```python
from build123d import *

# Parameters (mm, degrees)
SKETCH_1_R          = 45
SKETCH_1_R_2        = 2.6
SKETCH_1_R_3        = 35
EXTRUDE_2_DEPTH     = 5
EXTRUDE_START       = -5
SKETCH_3_R          = 47.8
SKETCH_3_R_2        = 45
EXTRUDE_3_DEPTH     = 5
CUT_EXTRUDE_1_DEPTH = 10


with BuildPart() as part:
    # 草图1 → 凸台-拉伸2 (new body)
    with BuildSketch(Plane.XY):
        Circle(SKETCH_1_R)
        with Locations((0, 40)):
            Circle(SKETCH_1_R_2, mode=Mode.SUBTRACT)
        with Locations((28.284271247, 28.284271247)):
            Circle(SKETCH_1_R_2, mode=Mode.SUBTRACT)
        with Locations((40, 0)):
            Circle(SKETCH_1_R_2, mode=Mode.SUBTRACT)
        with Locations((28.284271247, -28.284271247)):
            Circle(SKETCH_1_R_2, mode=Mode.SUBTRACT)
        with Locations((0, -40)):
            Circle(SKETCH_1_R_2, mode=Mode.SUBTRACT)
        with Locations((-28.284271247, -28.284271247)):
            Circle(SKETCH_1_R_2, mode=Mode.SUBTRACT)
        Circle(SKETCH_1_R_3, mode=Mode.SUBTRACT)
        with Locations((-40, 0)):
            Circle(SKETCH_1_R_2, mode=Mode.SUBTRACT)
        with Locations((-28.284271247, 28.284271247)):
            Circle(SKETCH_1_R_2, mode=Mode.SUBTRACT)
    extrude(amount=EXTRUDE_2_DEPTH)

    # 草图3 → 凸台-拉伸3 (add)
    with BuildSketch(Plane.XY.offset(5).offset(EXTRUDE_START)):
        Circle(SKETCH_3_R)
        Circle(SKETCH_3_R_2, mode=Mode.SUBTRACT)
    extrude(amount=EXTRUDE_3_DEPTH)

    # 草图4 → 切除-拉伸1 (cut)
    with BuildSketch(Plane.XY.offset(5)):
        with BuildLine():
            ThreePointArc((-8.473137213, 41.646799946), (-16.264045876, 39.264880132), (-23.457321876, 35.440147438))
            ThreePointArc((-23.457321876, 35.440147438), (-24.162193968, 31.975590419), (-20.697636949, 31.270718328))
            ThreePointArc((-20.697636949, 31.270718328), (-14.350628714, 34.645482469), (-7.476297541, 36.747176423))
            ThreePointArc((-7.476297541, 36.747176423), (-5.524905615, 39.695408021), (-8.473137213, 41.646799946))
        make_face()
        with BuildLine():
            ThreePointArc((23.457321876, 35.440147438), (16.264045876, 39.264880132), (8.473137213, 41.646799946))
            ThreePointArc((8.473137213, 41.646799946), (5.524905615, 39.695408021), (7.476297541, 36.747176423))
            ThreePointArc((7.476297541, 36.747176423), (14.350628714, 34.645482469), (20.697636949, 31.270718328))
            ThreePointArc((20.697636949, 31.270718328), (24.162193968, 31.975590419), (23.457321876, 35.440147438))
        make_face()
        with BuildLine():
            ThreePointArc((41.646799946, 8.473137213), (39.264880132, 16.264045876), (35.440147438, 23.457321876))
            ThreePointArc((35.440147438, 23.457321876), (31.975590419, 24.162193968), (31.270718328, 20.697636949))
            ThreePointArc((31.270718328, 20.697636949), (34.645482469, 14.350628714), (36.747176423, 7.476297541))
            ThreePointArc((36.747176423, 7.476297541), (39.695408021, 5.524905615), (41.646799946, 8.473137213))
        make_face()
        with BuildLine():
            ThreePointArc((35.440147438, -23.457321876), (39.264880132, -16.264045876), (41.646799946, -8.473137213))
            ThreePointArc((41.646799946, -8.473137213), (39.695408021, -5.524905615), (36.747176423, -7.476297541))
            ThreePointArc((36.747176423, -7.476297541), (34.645482469, -14.350628714), (31.270718328, -20.697636949))
            ThreePointArc((31.270718328, -20.697636949), (31.975590419, -24.162193968), (35.440147438, -23.457321876))
        make_face()
        with BuildLine():
            ThreePointArc((8.473137213, -41.646799946), (16.264045876, -39.264880132), (23.457321876, -35.440147438))
            ThreePointArc((23.457321876, -35.440147438), (24.162193968, -31.975590419), (20.697636949, -31.270718328))
            ThreePointArc((20.697636949, -31.270718328), (14.350628714, -34.645482469), (7.476297541, -36.747176423))
            ThreePointArc((7.476297541, -36.747176423), (5.524905615, -39.695408021), (8.473137213, -41.646799946))
        make_face()
        with BuildLine():
            ThreePointArc((-23.457321876, -35.440147438), (-16.264045876, -39.264880132), (-8.473137213, -41.646799946))
            ThreePointArc((-8.473137213, -41.646799946), (-5.524905615, -39.695408021), (-7.476297541, -36.747176423))
            ThreePointArc((-7.476297541, -36.747176423), (-14.350628714, -34.645482469), (-20.697636949, -31.270718328))
            ThreePointArc((-20.697636949, -31.270718328), (-24.162193968, -31.975590419), (-23.457321876, -35.440147438))
        make_face()
        with BuildLine():
            ThreePointArc((-41.646799946, -8.473137213), (-39.264880132, -16.264045876), (-35.440147438, -23.457321876))
            ThreePointArc((-35.440147438, -23.457321876), (-31.975590419, -24.162193968), (-31.270718328, -20.697636949))
            ThreePointArc((-31.270718328, -20.697636949), (-34.645482469, -14.350628714), (-36.747176423, -7.476297541))
            ThreePointArc((-36.747176423, -7.476297541), (-39.695408021, -5.524905615), (-41.646799946, -8.473137213))
        make_face()
        with BuildLine():
            ThreePointArc((-35.440147438, 23.457321876), (-39.264880132, 16.264045876), (-41.646799946, 8.473137213))
            ThreePointArc((-41.646799946, 8.473137213), (-39.695408021, 5.524905615), (-36.747176423, 7.476297541))
            ThreePointArc((-36.747176423, 7.476297541), (-34.645482469, 14.350628714), (-31.270718328, 20.697636949))
            ThreePointArc((-31.270718328, 20.697636949), (-31.975590419, 24.162193968), (-35.440147438, 23.457321876))
        make_face()
    extrude(amount=-CUT_EXTRUDE_1_DEPTH, mode=Mode.SUBTRACT)


solid = part.part
```
Could you check a few things on this model? Use its own coordinates, in mm. A direction names the side the tool comes from. Round coordinates to 2 decimals unless told otherwise and drop trailing zeros. Write each loop counter-clockwise with the first axis right and the second up, starting at its lowest first coordinate (ties: lowest second). Pieces come first, ordered by that corner, then holes. Notation, with made-up numbers: M 24,-13 L 30,-13 A10 cw 30,-5 Z; hole C 34,31 d2. An arc over 180 degrees is marked long. Answer in a Markdown table with one row per item. Add a question column.
Q1. If we mould it in two halves opening along X, with no side actions, what happens to faces 3 (the flat face through (0, 36, 0)), 4 (the cylindrical face through (39.641, 5.515, 2.535))? For each: +X half, -X half, draft (parallel to the pull), parting line (faces both ways), or undercut.
Q2. On a 3-axis mill with a long thin cutter (end or side, diameter ignored), from which of +Z, -Z, +X, -X, +Y, -Y can I reach the whole of each face in a straight line? I mean faces 1 (the flat face through (0, 36, 5)), 2 (the cylindrical face through (-39.22, 16.37, 2.54)). Say none if no direction works.
Q3. Imagine slicing it at A-A (x = 0). Please give me the cut outline in (y, z).
Q4. Will these pins go through, and if not, where does the flat tip stop? pin 1 Ø3 at (x, z) = (12, 2.5) entering from -Y; pin 2 Ø2 at (y, z) = (32, 1) entering from +X; pin 3 Ø2 at (x, z) = (7, 2) entering from +Y.
Q5. If I drill on line 1 (Y direction, x = 0, z = 1.8); line 2 (Y direction, x = 16.5, z = 2.35); line 3 (X direction, y = 24, z = 3.05), over which ranges is the centre line in solid material (lowest first)? Write a range as from..to.
Q6. Imagine slicing it at C-C (z = 1.75). Give the number of separate pieces and of enclosed holes in the cut face, then the cut area to 3 significant figures.
Values:
| question | item | result |
|---|---|---|
| 1 | face 3 | draft |
| 1 | face 4 | undercut |
| 2 | face 1 | +Z, +X, -X, +Y, -Y |
| 2 | face 2 | +Z, -Z |
| 3 | outline | M -47.8,0 L -42.6,0 L -42.6,5 L -47.8,5 Z; M -37.4,0 L -35,0 L -35,5 L -37.4,5 Z; M 35,0 L 37.4,0 L 37.4,5 L 35,5 Z; M 42.6,0 L 47.8,0 L 47.8,5 L 42.6,5 Z |
| 4 | pin 1 | y = -46.63 |
| 4 | pin 2 | x = 36.38 |
| 4 | pin 3 | y = 47.42 |
| 5 | line 1 | -47.8..-42.6, -37.4..-35, 35..37.4, 42.6..47.8 |
| 5 | line 2 | -44.86..-39.17, -33.67..-30.87, 30.87..33.67, 39.17..44.86 |
| 5 | line 3 | -41.34..-34.95, -31.76..-25.48, 25.48..31.76, 34.95..41.34 |
| 6 | separate pieces | 1 |
| 6 | enclosed holes | 17 |
| 6 | area | 2,390 mm^2 |
